```python
from build123d import *

# Parameters (mm, degrees)
SKETCH1_R           = 1.5
SKETCH1_R_2         = 1
SKETCH1_R_3         = 2.5
BOSS_EXTRUDE1_DEPTH = 2


with BuildPart() as part:
    # Sketch1 → Boss-Extrude1 (new body)
    with BuildSketch(Plane(origin=(0, 0, 0), x_dir=(1, 0, 0), z_dir=(0, 1, 0))):
        Polygon((-125, -50), (-60, -100.598017019), (60, -100.598017019), (125, -50), (125, 99.401982981), (-125, 99.401982981), align=None)
        with Locations(Location((-77.896249371, 49.467404951, 0), (0, 0, 270))):
            Circle(SKETCH1_R, mode=Mode.SUBTRACT)
        with Locations(Location((-77.896249371, 79.467404951, 0), (0, 0, 270))):
            Circle(SKETCH1_R, mode=Mode.SUBTRACT)
        with Locations(Location((-113.896249371, 79.467404951, 0), (0, 0, 270))):
            Circle(SKETCH1_R, mode=Mode.SUBTRACT)
        with Locations(Location((-113.896249371, 49.467404951, 0), (0, 0, 270))):
            Circle(SKETCH1_R, mode=Mode.SUBTRACT)
        with Locations(Location((113.896249371, 49.467404951, 0), (0, 0, 270))):
            Circle(SKETCH1_R, mode=Mode.SUBTRACT)
        with Locations(Location((113.896249371, 79.467404951, 0), (0, 0, 270))):
            Circle(SKETCH1_R, mode=Mode.SUBTRACT)
        with Locations(Location((77.896249371, 79.467404951, 0), (0, 0, 270))):
            Circle(SKETCH1_R, mode=Mode.SUBTRACT)
        with Locations(Location((77.896249371, 49.467404951, 0), (0, 0, 270))):
            Circle(SKETCH1_R, mode=Mode.SUBTRACT)
        with Locations(Location((-18, 81.850418852, 0), (0, 0, 270))):
            Circle(SKETCH1_R_2, mode=Mode.SUBTRACT)
        with Locations(Location((-18, 45.850418852, 0), (0, 0, 270))):
            Circle(SKETCH1_R_2, mode=Mode.SUBTRACT)
        with Locations(Location((18, 81.850418852, 0), (0, 0, 270))):
            Circle(SKETCH1_R_2, mode=Mode.SUBTRACT)
        with Locations(Location((18, 45.850418852, 0), (0, 0, 270))):
            Circle(SKETCH1_R_2, mode=Mode.SUBTRACT)
        with Locations(Location((-12, -59.472750438, 0), (0, 0, 270))):
            Circle(SKETCH1_R_3, mode=Mode.SUBTRACT)
        with Locations(Location((12, -59.472750438, 0), (0, 0, 270))):
            Circle(SKETCH1_R_3, mode=Mode.SUBTRACT)
        with Locations(Location((12, -89.472750438, 0), (0, 0, 270))):
            Circle(SKETCH1_R_3, mode=Mode.SUBTRACT)
        with Locations(Location((-12, -89.472750438, 0), (0, 0, 270))):
            Circle(SKETCH1_R_3, mode=Mode.SUBTRACT)
        Polygon((-69.896249371, 32.980170885), (-69.896249371, 28.980170885), (-73.896249371, 28.980170885), (-73.896249371, 24.980170885), (-77.896249371, 24.980170885), (-77.896249371, 32.980170885), align=None, mode=Mode.SUBTRACT)
        Polygon((-77.896249371, -24.980170885), (-77.896249371, -32.980170885), (-69.896249371, -32.980170885), (-69.896249371, -28.980170885), (-73.896249371, -28.980170885), (-73.896249371, -24.980170885), align=None, mode=Mode.SUBTRACT)
        Polygon((79.650184211, 32.980170885), (87.650184211, 32.980170885), (87.650184211, 24.980170885), (83.650184211, 24.980170885), (83.650184211, 28.980170885), (79.650184211, 28.980170885), align=None, mode=Mode.SUBTRACT)
        Polygon((83.650184211, -28.980170885), (79.650184211, -28.980170885), (79.650184211, -32.980170885), (87.650184211, -32.980170885), (87.650184211, -24.980170885), (83.650184211, -24.980170885), align=None, mode=Mode.SUBTRACT)
    extrude(amount=BOSS_EXTRUDE1_DEPTH)


solid = part.part
```
Work out the finished part from the listing and answer in its coordinate system (mm). Give positions to 0.01 mm unless a question says otherwise; leave off trailing zeros. Loops run counter-clockwise (first coordinate to the right, second up) from the corner with the lowest first, then second, coordinate; pieces in that order, holes last. Notation, with made-up numbers: (18, 46) - (63, 46) arc R18 ccw to (63, 76) - close; hole circle Ø4 at (60.25, -5.75). An arc over 180 degrees is marked (long way). One line per question, with ' | ' between items.
(1) Each of these flat-tipped pins is pushed along its axis until it touches: pin 1 Ø1 at (x, y) = (85.5, 1) entering from +Z; pin 2 Ø8 at (x, z) = (-12, 89.47) entering from +Y; pin 3 Ø0.6 at (x, y) = (82, 1) entering from +Z. Where does it stop, or does it pass through?
Recorded:
pin 1: stops at z = 81.14 | pin 2: stops at y = 2 | pin 3: stops at z = 83.71
(2) The part is cut by section B-B (z = 80). Write down the section's boundary in (x, y).
Recorded:
outline: (-86.46, 0) - (86.46, 0) - (86.46, 2) - (-86.46, 2) - close
(3) The mould has two halves that part along X. Classify faces 1 (the face through (-14.218, 0.986, 90.626)), 2 (the face through (92.045, 0.986, 75.653)), 3 (the face through (-2, 0, -1)): +X half, -X half, draft (parallel to the pull), parting line (faces both ways), or undercut.
Recorded:
face 1: undercut | face 2: +X half | face 3: draft
(4) The part is cut by section A-A (y = 1.7). Count the separate pieces of the cut face and the enclosed holes in it, then the cut area to 3 significant figures.
Recorded:
separate pieces: 1 | enclosed holes: 20 | area: 46,400 mm²
(5) Straight lines are drawn through the part: probe 1 along X at (y, z) = (1.95, -27); probe 2 along X at (y, z) = (1.85, -50.5); probe 3 along X at (y, z) = (1, -46). For each, find the intervals that lie inside material, in ascending order.
Recorded:
probe 1: x = -125 to -77.9, -73.9 to 83.65, 87.65 to 125 | probe 2: x = -125 to -114.98, -112.81 to -78.98, -76.81 to 76.81, 78.98 to 112.81, 114.98 to 125 | probe 3: x = -125 to -18.99, -17.01 to 17.01, 18.99 to 125
